Here's the drawing with two shaded views (mm, measured from the low corner). I have some questions. A direction names the side the tool comes from. Coordinates: 2 decimals unless noted, no trailing zeros. Loops run counter-clockwise (first coordinate to the right, second up) from the corner with the lowest first, then second, coordinate; pieces in that order, holes last.
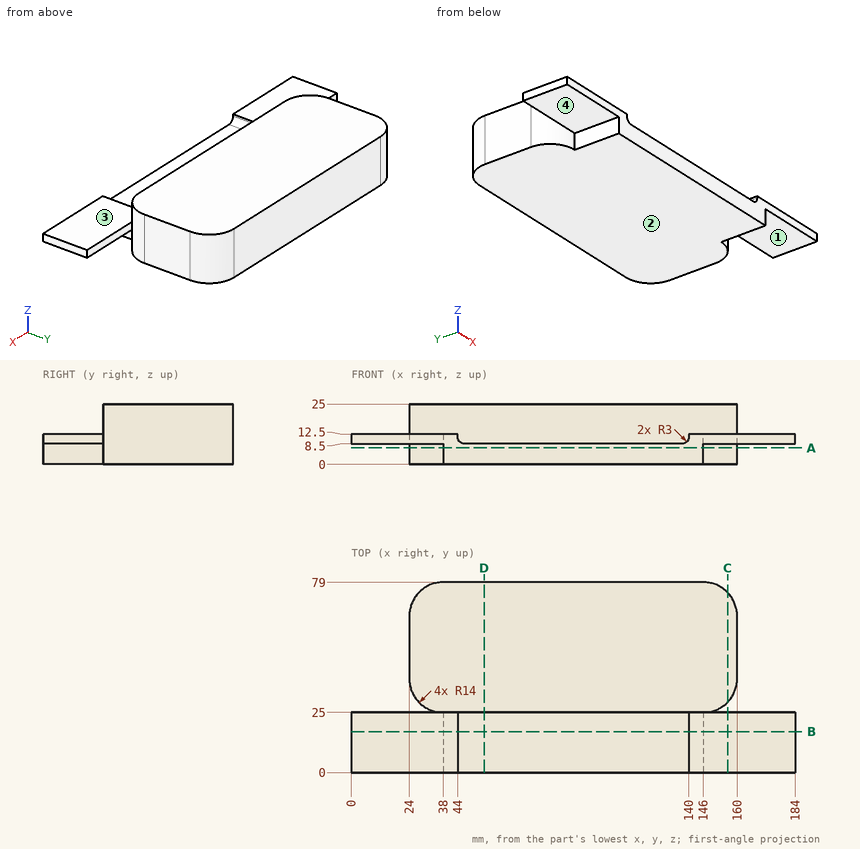
(1) I want a section at A-A on z = 6.75. Write out the boundary of the cut face in (x, y).
Check values:
outline: (24, 39) arc R14 ccw to (38, 25) - (38, 0) - (146, 0) - (146, 25) arc R14 ccw to (160, 39) - (160, 65) arc R14 ccw to (146, 79) - (38, 79) arc R14 ccw to (24, 65) - close
(2) I'm going to push flat-ended pins straight in: pin 1 (20 mm diameter, centred on x = 161.5, y = 14.5, fed in from +Z); pin 2 (1.2 mm diameter, centred on x = 172.5, z = 9.5, fed in from +Y); pin 3 (0.8 mm diameter, centred on y = 10.5, z = 12, fed in from -X); pin 4 (20 mm diameter, centred on x = 160.5, y = 13.5, fed in from -Z). Where does each tip first touch, or does it pass through?
Check values:
pin 1: stops at z = 12.5
pin 2: stops at y = 25
pin 3: stops at x = 0
pin 4: stops at z = 8.5
(3) I want a section at C-C on x = 156. Write out the boundary of the cut face in (y, z).
Check values:
outline: (0, 8.5) - (25, 8.5) - (25, 12.5) - (0, 12.5) - close; (29.2, 0) - (74.8, 0) - (74.8, 25) - (29.2, 25) - close
(4) I want a section at D-D on x = 55. Write out the boundary of the cut face in (y, z).
Check values:
outline: (0, 0) - (79, 0) - (79, 25) - (25, 25) - (25, 8.5) - (0, 8.5) - close
(5) Which directions (+Z, -Z, +X, -X, +Y, -Y) give clear straight access to the entire face, cutting with the end or side of a thin tool? Please do the marked faces 1, 2, 3 and 4.
Check values:
face 1: -Z, +X, -Y
face 2: -Z, +X, -X, +Y, -Y
face 3: +Z, +X, -X, -Y
face 4: -Z, -X, -Y
(6) I want a section at B-B on y = 17. Write out the boundary of the cut face in (x, z), then the cut area to 3 significant figures.
Check values:
outline: (0, 8.5) - (38, 8.5) - (38, 0) - (146, 0) - (146, 8.5) - (184, 8.5) - (184, 12.5) - (140, 12.5) - (140, 11.5) arc R3 cw to (137, 8.5) - (47, 8.5) arc R3 cw to (44, 11.5) - (44, 12.5) - (0, 12.5) - close
area: 1,270 mm2
(7) If I drill on probe 1 along Y at (x, z) = (102.5, 9.5); probe 2 along Z at (x, y) = (18, 14); probe 3 along X at (y, z) = (58, 22.5), over which ranges is the centre line in solid material (lowest first)?
Check values:
probe 1: y = 25 to 79
probe 2: z = 8.5 to 12.5
probe 3: x = 24 to 160
